Work out the finished part from the listing and answer in its coordinate system (mm). A direction names the side the tool comes from. Round coordinates to 2 decimals unless told otherwise and drop trailing zeros. Order: outer loops, then holes, each group sorted by start corner. A loop starts at its lowest first (then second) coordinate and runs counter-clockwise, first axis right, second up. Notation, with made-up numbers: (68, 54.25) - (97, 54.25) arc R25 ccw to (97, 75.25) - close; hole circle Ø4 at (-3, 80.5). An arc over 180 degrees is marked (long way). Use CSV: the item, a comma, the result in double quotes.
Autodesk Inventor part; units mm, degrees
ref_plane "YZ Plane" through (0, 0, 0) normal (1, 0, 0) x (0, 1, 0)
ref_plane "XZ Plane" through (0, 0, 0) normal (0, 1, 0) x (-1, 0, 0)
ref_plane "XY Plane" through (0, 0, 0) normal (0, 0, 1) x (1, 0, 0)
sketch "Sketch1" plane through (0, 0, 0) normal (1, 0, 0) x (0, 1, 0)
  line L0 (330.216, 0) -> (0, 0)
  line L1 (0, 0) -> (0, 164.8957)
  arc A0 (118.7293, 313.7601) -> (0, 164.8957) centre (156.123, 162.1567) ccw
  arc A1 (144.8949, 317.2465) -> (118.7293, 313.7601) centre (154.9782, 141.6407) ccw
  line L2 (144.8949, 317.2465) -> (181.2781, 317.4432)
  arc A2 (330.216, 164.8957) -> (181.2781, 317.4432) centre (176.28, 163.5828) ccw
  line L3 (330.216, 164.8957) -> (330.216, 0)
  line L4 (330.216, 0) -> (0, 0)
  arc A3 (290.5507, 48.5961) -> (284.7281, 100.708) centre (242.7487, 69.6363) ccw
  circle A4 centre (242.7487, 69.6363) radius 50
  arc A5 (57.0662, 113.5176) -> (48.9146, 32.5841) centre (90.2937, 69.2937) ccw
  circle A6 centre (90.2937, 69.2937) radius 50
  circle A7 centre (165.108, 261.7017) radius 20
  dimension "d0" = 100
  dimension "d1" = 100
  dimension "d2" = 40
sketch "Sketch2" plane through (0, 0, 0) normal (0, 1, 0) x (-1, 0, 0)
  line L0 (-2089.1825, 1088.7803) -> (2413.4361, 1088.7803)
  line L1 (2413.4361, 1088.7803) -> (2413.4361, -1008.0732)
  line L2 (2413.4361, -1008.0732) -> (-2089.1825, -1008.0732)
  line L3 (-2089.1825, -1008.0732) -> (-2089.1825, 1088.7803)
  line L4 (-994.3855, 154.3994) -> (-877.0981, 0)
  line L5 (-877.0981, 0) -> (-549.3425, 0)
  line L6 (-549.3425, 0) -> (-549.3425, 138.7482)
  line L7 (-549.3425, 138.7482) -> (-727.3007, 309.2752)
  line L8 (-727.3007, 309.2752) -> (-869.8451, 302.5626)
  line L9 (-869.8451, 302.5626) -> (-881.5787, 366.7057)
  arc A0 (-869.8451, 302.5626) -> (-994.3855, 154.3994) centre (-863.6463, 170.9285) ccw
  line L10 (-172.1358, 318.294) -> (-272.072, 318.294)
  line L11 (-272.072, 318.294) -> (-450.7939, 141.6872)
  line L12 (-450.7939, 141.6872) -> (-450.7939, 0)
  line L13 (-450.7939, 0) -> (3.9431, 0)
  line L14 (3.9431, 0) -> (3.9431, 140.1064)
  line L15 (3.9431, 140.1064) -> (-172.1358, 318.294)
  line L16 (98.5967, 142.2155) -> (98.5967, 0)
  line L17 (98.5967, 0) -> (660.1371, 0)
  line L18 (660.1371, 0) -> (660.1371, 140.1064)
  line L19 (660.1371, 140.1064) -> (484.0582, 318.294)
  line L20 (484.0582, 318.294) -> (276.784, 318.294)
  line L21 (276.784, 318.294) -> (98.5967, 142.2155)
  point P0 (0, 0)
extrude "Extrusion1" add sketch "Sketch1" along normal mid plane 3000
extrude "Extrusion2" cut sketch "Sketch2" along normal mid plane 3000
sketch "Sketch3" plane through (0, 0, 0) normal (0, 0, 1) x (1, 0, 0)
  line L0 (-659.4013, 331.8291) -> (-659.4013, 0)
  line L1 (-659.4013, 0) -> (-101.5785, 2.8306)
  line L2 (-101.5785, 2.8306) -> (-101.5785, 327.2485)
  line L3 (-101.5785, 327.2485) -> (-659.4013, 331.8291)
  line L4 (-6.3615, 322.7102) -> (-6.3615, 2.311)
  line L5 (-6.3615, 2.311) -> (451.0837, 8.3992)
  line L6 (451.0837, 8.3992) -> (451.0837, 322.7102)
  line L7 (451.0837, 322.7102) -> (-6.3615, 322.7102)
  line L8 (550.0381, 321.2751) -> (550.0381, 9.7162)
  line L9 (550.0381, 9.7162) -> (880.8921, 11.9316)
  line L10 (880.8921, 11.9316) -> (881.9732, 8.1918)
  line L11 (550.0381, 321.2751) -> (881.436, 318.556)
  line L12 (881.436, 318.556) -> (884.7001, 327.2485)
  arc A0 (994.4459, 201.1298) -> (881.436, 318.556) centre (879.2692, 203.3778) ccw
  arc A1 (880.8921, 11.9316) -> (994.4459, 129.9671) centre (880.1263, 126.3072) ccw
  line L13 (994.4459, 201.1298) -> (994.4459, 129.9671)
  line L14 (-921.3329, 565.6411) -> (1466.6724, 565.6411)
  line L15 (1466.6724, 565.6411) -> (1466.6724, -337.8722)
  line L16 (1466.6724, -337.8722) -> (-921.3329, -337.8722)
  line L17 (-921.3329, -337.8722) -> (-921.3329, 565.6411)
  point P0 (0, 0)
extrude "Extrusion3" cut sketch "Sketch3" along normal mid plane 3000
chamfer_without_effect "Chamfer1"
sketch "Sketch5" plane through (-659.4013, 0, 0) normal (0, 0, -1) x (-1, 0, 0)
  line L0 (117.9817, -138.9278) -> (-593.002, -138.9278)
  line L1 (-593.002, -138.9278) -> (-593.002, 563.8836)
  line L2 (-593.002, 563.8836) -> (117.9817, 563.8836)
  line L3 (117.9817, 563.8836) -> (117.9817, -138.9278)
  line L4 (-1175.2731, -102.1528) -> (-1759.5873, -102.1528)
  line L5 (-1759.5873, -102.1528) -> (-1759.5873, 529.1516)
  line L6 (-1759.5873, 529.1516) -> (-1175.2731, 529.1516)
  line L7 (-1175.2731, 529.1516) -> (-1175.2731, -102.1528)
  point P0 (-659.4013, 0)
extrude "Extrusion5" cut sketch "Sketch5" along normal mid plane 2000
move faces "Move1" translate (250, 0, 0) faces at (450.7939, 188.0332, 134.0166) (417.0556, 165.298, 175.0262)
sketch "Sketch6" plane through (-3.9431, 2.3432, 0) normal (0, 0, -1) x (-1, 0, 0)
  circle A0 centre (-681.7661, 301.457) radius 11.0515
  line L0 (-704.737, 290.4055) -> (0, 290.4055)
  line L1 (-160.9181, 269.1956) -> (-345.3885, 269.1956)
  line L2 (-345.3885, 269.1956) -> (-345.3885, 246.2614)
  line L3 (-345.3885, 246.2614) -> (-160.9181, 246.2614)
  line L4 (-160.9181, 246.2614) -> (-160.9181, 269.1956)
  line L5 (-237.6977, 269.1956) -> (-160.9181, 175.4646)
  line L6 (-160.9181, 175.4646) -> (-179.8547, 159.9527)
  line L7 (-179.8547, 159.9527) -> (-256.6343, 253.6837)
  line L8 (-256.6343, 253.6837) -> (-237.6977, 269.1956)
  line L9 (-256.6343, 253.6837) -> (-282.5689, 261.4396)
  line L10 (-282.5689, 261.4396) -> (-309.0263, 172.9706)
  line L11 (-309.0263, 172.9706) -> (-283.0918, 165.2146)
  line L12 (-283.0918, 165.2146) -> (-256.6343, 253.6837)
  point P0 (-3.9431, -2.3432)
  point P1 (-287.108, 246.2614)
  point P2 (-258.854, 246.2614)
  point P3 (-250.5544, 246.2614)
  point P4 (-218.9112, 246.2614)
extrude "Extrusion6" cut sketch "Sketch6" against normal blind 5
properties part number "Kleiner Finger middle"
(1) Find the intervals of material crossed by L1, parallel to Y at x = 222, z = 67; L2, parallel to Y at x = 501.5, z = 101; L3, parallel to Z at x = 118, y = 49, in increasing order. Write a range as from..to.
Findings below:
L1,"y = 5.35..40.35, 140.24..192.82, 292.68..322.71"
L2,"y = 9.07..51.63, 128.96..203.81, 281.69..322.71"
L3,"z = 0..41.1, 97.49..263.51"
(2) Find section C-C (x = 369). Determine the outline of the cut face in (y, z).
Findings below:
outline,"(7.31, 0) - (322.71, 0) - (322.71, 211.08) arc R153.94 ccw to (181.28, 317.44) - (144.89, 317.25) arc R175.9 ccw to (118.73, 313.76) arc R156.15 ccw to (7.31, 209.44) - close; hole circle Ø100 at (90.29, 69.29); hole circle Ø40 at (165.11, 261.7); hole circle Ø100 at (242.75, 69.64)"
(3) Find section A-A (y = 89). Determine the outline of the cut face in (x, z).
Findings below:
outline,"(-3.94, 0) - (700.79, 0) - (700.79, 19.31) - (-3.94, 19.31) - close; (-3.94, 119.28) - (700.79, 119.28) - (700.79, 141.69) - (537.41, 303.14) - (157.16, 303.14) - (-3.94, 140.11) - close"
(4) Each of these flat-tipped pins is pushed along its axis until it touches: pin 1 (5.5 mm diameter, centred on x = 272.5, z = 3.5, fed in from -Y); pin 2 (3 mm diameter, centred on x = 379, y = 267.5, fed in from +Z); pin 3 (2 mm diameter, centred on x = 87, y = 138.5, fed in from -Z); pin 4 (2 mm diameter, centred on y = 118.5, z = 193, fed in from -X). Where does it stop, or does it pass through?
Findings below:
pin 1,"stops at y = 5.99"
pin 2,"stops at z = 288.68"
pin 3,"stops at z = 0"
pin 4,"stops at x = 47.34"
(5) Find section B-B (z = 89). Determine the outline of the cut face in (x, y), and give its area (3 significant figures).
Findings below:
outline,"(-3.94, 2.34) - (700.79, 11.72) - (700.79, 44.34) - (-3.94, 44.34) - close; (-3.94, 136.25) - (700.79, 136.25) - (700.79, 196.65) - (-3.94, 196.65) - close; (-3.94, 288.85) - (700.79, 288.85) - (700.79, 322.71) - (-3.94, 322.71) - close"
area,"92,700 mm²"
(6) For faces 1 (the flat face through (267.2, 207.51, 2.46)), 2 (the cylindrical face through (344.64, 131.56, 315.97)), determine the directions among +Z, -Z, +X, -X, +Y, -Y from which every point of the face is accessible in a straight line to the end or side of a thin tool.
Findings below:
face 1,"-Z"
face 2,"+Z, +X, -X, -Y"
(7) Find section D-D (y = 202). Determine the outline of the cut face in (x, z).
Findings below:
outline,"(-3.94, 0) - (176.79, 0) - (176.79, 5) - (208.44, 5) - (208.44, 0) - (268.85, 0) - (268.85, 5) - (297.1, 5) - (297.1, 0) - (700.79, 0) - (700.79, 40.66) - (-3.94, 40.66) - close; (-3.94, 98.61) - (700.79, 98.61) - (700.79, 141.69) - (525.04, 315.36) - (169.24, 315.36) - (-3.94, 140.11) - close"
(8) The mould has two halves that part along Z. Classify faces 3 (the flat face through (700.794, 165, 72)), 4 (the cylindrical face through (343.5, 203.1, 100.1)), 5 (the flat face through (678, 304, 5)), 6 (the cylindrical face through (344.494, 162.504, 241.872)): released by +Z, released by -Z, zero draft, split by the parting line, or undercut.
Findings below:
face 3,"zero draft"
face 4,"undercut"
face 5,"released by -Z"
face 6,"undercut"
